Check sheet for the modelled part. Datum: model origin and axes. Units: mm. A direction names the side the tool comes from. Coordinates: 2 decimals unless noted, no trailing zeros. Loops run counter-clockwise (first coordinate to the right, second up) from the corner with the lowest first, then second, coordinate; pieces in that order, holes last. Notation, with made-up numbers: (43.25, 35) -> (92.25, 35) arc R17 ccw to (92.25, 64) -> close; hole circle Ø1 at (60.5, 13.25). An arc over 180 degrees is marked (long way). Use one line per item in the form item = value.
from build123d import *

# Parameters (mm, degrees)
EXTRUDE_2_DEPTH     = 100
SKETCH_8_R          = 355
SKETCH_8_R_2        = 275
CUT_EXTRUDE_1_DEPTH = 5
CUT_EXTRUDE_2_DEPTH = 5
CUT_EXTRUDE_3_DEPTH = 5
SKETCH_13_W         = 100
SKETCH_13_H         = 932.842712474
EXTRUDE_3_DEPTH     = 900


with BuildPart() as part:
    # 草图2 → 凸台-拉伸2 (new body)
    with BuildSketch(Plane(origin=(0, 0, 0), x_dir=(1, 0, 0), z_dir=(0, 1, 0))):
        Polygon((-425, 750), (425, 750), (750, 425), (750, -425), (425, -750), (-425, -750), (-750, -425), (-750, 425), align=None)
    extrude(amount=EXTRUDE_2_DEPTH)

    # 草图4 → 放样4 section 0
    with BuildSketch(Plane.XZ):
        Polygon((-466.421356237, 850), (466.421356237, 850), (850, 466.421356237), (850, -466.421356237), (466.421356237, -850), (-466.421356237, -850), (-850, -466.421356237), (-850, 466.421356237), align=None)
    # 草图7 → 放样4 section 1
    with BuildSketch(Plane(origin=(0, 50, 0), x_dir=(1, 0, 0), z_dir=(0, 1, 0))):
        Polygon((750, -425), (425, -750), (-425, -750), (-750, -425), (-750, 425), (-425, 750), (425, 750), (750, 425), align=None)
    loft()

    # 草图8 → 切除-拉伸1 (cut)
    with BuildSketch(Plane(origin=(0, 100, 0), x_dir=(1, 0, 0), z_dir=(0, 1, 0))):
        Circle(SKETCH_8_R)
        Circle(SKETCH_8_R_2, mode=Mode.SUBTRACT)
    extrude(amount=-CUT_EXTRUDE_1_DEPTH, mode=Mode.SUBTRACT)

    # 草图9 → 切除-拉伸2 (cut)
    with BuildSketch(Plane(origin=(0, 100, 0), x_dir=(1, 0, 0), z_dir=(0, 1, 0))):
        Polygon((-196.260530097, 136.438578222), (203.739469903, 136.438578222), (203.739469903, 86.438578222), (28.739469903, 86.438578222), (28.739469903, -86.438578222), (203.739469903, -86.438578222), (203.739469903, -136.438578222), (-196.260530097, -136.438578222), (-196.260530097, -86.438578222), (-21.260530097, -86.438578222), (-21.260530097, 86.438578222), (-196.260530097, 86.438578222), align=None)
    extrude(amount=-CUT_EXTRUDE_2_DEPTH, mode=Mode.SUBTRACT)

    # 草图10 → 切除-拉伸3 (cut)
    with BuildSketch(Plane(origin=(0, 100, 0), x_dir=(1, 0, 0), z_dir=(0, 1, 0))):
        Polygon((425, 750), (-425, 750), (-750, 425), (-750, -425), (-425, -750), (425, -750), (750, -425), (750, 425), align=None)
        Polygon((700, 404.289321881), (700, -404.289321881), (404.289321881, -700), (-404.289321881, -700), (-700, -404.289321881), (-700, 404.289321881), (-404.289321881, 700), (404.289321881, 700), align=None, mode=Mode.SUBTRACT)
    extrude(amount=-CUT_EXTRUDE_3_DEPTH, mode=Mode.SUBTRACT)

    # 草图13 → 凸台-拉伸3 (add)
    with BuildSketch(Plane.XZ):
        with Locations((-800, 0)):
            Rectangle(SKETCH_13_W, SKETCH_13_H)
        with Locations((800, 0)):
            Rectangle(SKETCH_13_W, SKETCH_13_H)
    extrude(amount=EXTRUDE_3_DEPTH)


solid = part.part
(1) Tool access check on faces 4 (the flat face through (550.075, 97.535, -554.215)), 5 (the flat face through (799, -444, 466.421)), 6 (the flat face through (-550.075, 97.535, 554.215)). Record the directions out of +Z, -Z, +X, -X, +Y, -Y that give a thin tool (end or side, any length) a straight path to the whole face; none if there is none.
Established:
face_4 = -Z, +X, +Y
face_5 = +Z, +X, -X, -Y
face_6 = +Z, -X, +Y
(2) Go/stop test with flat-tipped pins: P1, Ø2.5, axis at y = 96.5, z = -106, coming from the +X side; P2, Ø5.5, axis at y = 98.5, z = 120.5, coming from the -X side; P3, Ø22.5, axis at x = 192, y = 64, coming from the -Z side. Record where each tip stops, or that it passes through.
Established:
P1 = 700
P2 = -700
P3 = -750
(3) Scan lines: line 1 along Z through (x, y) = (0, 97.3); line 2 along X through (y, z) = (96.75, 0); line 3 along X through (y, z) = (-552, -432.5). Record each from-to range of solid material in increasing order.
Established:
line_1 = -700 to -355, -275 to -136.44, 136.44 to 275, 355 to 700
line_2 = -700 to -355, -275 to -21.26, 28.74 to 275, 355 to 700
line_3 = -850 to -750, 750 to 850
(4) Section check A-A, the plane y = -275. Record the boundary of the cut face in (x, z), plus the area to 3 significant figures.
Established:
outline = (-850, -466.42) -> (-750, -466.42) -> (-750, 466.42) -> (-850, 466.42) -> close; (750, -466.42) -> (850, -466.42) -> (850, 466.42) -> (750, 466.42) -> close
area = 187,000 mm²
(5) Mould release check, pull along X, two halves, no side actions. Record for faces 1 (the flat face through (5, 0, 18)), 2 (the flat face through (750, 72, -6)), 3 (the flat face through (-850, -444, -7)): +X half, -X half, draft (parallel to the pull), parting line (faces both ways), or undercut.
Established:
face_1 = undercut
face_2 = +X half
face_3 = -X half
